Design review of the part built by this model. Coordinates are the model's own, in mm. Give positions to 0.01 mm unless a question says otherwise; leave off trailing zeros. Write each loop counter-clockwise with the first axis right and the second up, starting at its lowest first coordinate (ties: lowest second). Pieces come first, ordered by that corner, then holes. Notation, with made-up numbers: M 0.25,2 L 57.25,2 A25 cw 57.25,25 Z; hole C 36,68 d10. An arc over 180 degrees is marked long. Use a Markdown table: item, result. Add a question column.
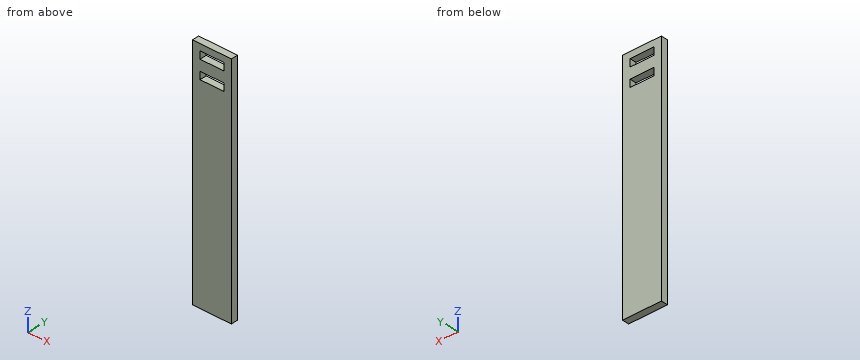
```python
from build123d import *

# Parameters (mm, degrees)
F0_W     = 11
F0_H     = 3.5
F0_W_2   = 3.5
F1_DEPTH = 3.2


with BuildPart() as f1:
    # F0 (on Front) → F1 (new body)
    with BuildSketch(Plane.XZ):
        Polygon((12.312121, 101.111746), (-5.687879, 101.111746), (-5.687879, 89.611746), (-2.187879, 89.611746), (8.812121, 89.611746), (12.312121, 89.611746), align=None)
        with Locations((3.312121, 96.361746)):
            Rectangle(F0_W, F0_H, mode=Mode.SUBTRACT)
        Polygon((-2.187879, 86.111746), (-5.687879, 86.111746), (-5.687879, -8.888254), (12.312121, -8.888254), (12.312121, 86.111746), (8.812121, 86.111746), align=None)
        with Locations((10.562121, 87.861746)):
            Rectangle(F0_W_2, F0_H)
        with Locations((-3.937879, 87.861746)):
            Rectangle(F0_W_2, F0_H)
    extrude(amount=-F1_DEPTH)


solid = f1.part
```
(1) Wall thickness on L1, parallel to Z at x = 8, y = 0.45; L2, parallel to X at y = 2.65, z = 89: over which ranges is each line inside the solid? List them lowest first.
(2) Add section A-A on x = 3. Give the boundary of the cut face in (y, z).
(3) Add section B-B on y = 0.55. Give the boundary of the cut face in (x, z), then the cut area to 3 significant figures.
From the geometry:
| question | item | result |
|---|---|---|
| 1 | L1 | z = -8.89 to 86.11, 89.61 to 94.61, 98.11 to 101.11 |
| 1 | L2 | x = -5.69 to -2.19, 8.81 to 12.31 |
| 2 | outline | M 0,-8.89 L 3.2,-8.89 L 3.2,86.11 L 0,86.11 Z; M 0,89.61 L 3.2,89.61 L 3.2,94.61 L 0,94.61 Z; M 0,98.11 L 3.2,98.11 L 3.2,101.11 L 0,101.11 Z |
| 3 | outline | M -5.69,-8.89 L 12.31,-8.89 L 12.31,101.11 L -5.69,101.11 Z; hole M -2.19,86.11 L 8.81,86.11 L 8.81,89.61 L -2.19,89.61 Z; hole M -2.19,94.61 L 8.81,94.61 L 8.81,98.11 L -2.19,98.11 Z |
| 3 | area | 1,900 mm^2 |
